from build123d import *

# Parameters (mm, degrees)
F1_DEPTH = 25


with BuildPart() as f1:
    # F0 (on Top) → F1 (new body)
    with BuildSketch(Plane.XY):
        with BuildLine():
            ThreePointArc((-37.094474, -66.332496), (-76, 0), (-37.094474, 66.332496))
            Line((-37.094474, 66.332496), (-37.094474, 82))
            ThreePointArc((-37.094474, 82), (-75.625732, 48.792916), (-90, 0))
            ThreePointArc((-90, 0), (-75.625732, -48.792916), (-37.094474, -82))
            Line((-37.094474, -82), (-37.094474, -66.332496))
        make_face()
        with BuildLine():
            ThreePointArc((-90, 0), (-75.625732, 48.792916), (-37.094474, 82))
            Line((-37.094474, 82), (-90, 82))
            Line((-90, 82), (-90, 0))
        make_face()
        with BuildLine():
            Line((-90, -82), (-37.094474, -82))
            ThreePointArc((-37.094474, -82), (-75.625732, -48.792916), (-90, 0))
            Line((-90, 0), (-90, -82))
        make_face()
    extrude(amount=F1_DEPTH)


solid = f1.part
Read the model definition and answer for the solid it produces. Units are mm, in the model's axes. Coordinates: 2 decimals unless noted, no trailing zeros. Order: outer loops, then holes, each group sorted by start corner. A loop starts at its lowest first (then second) coordinate and runs counter-clockwise, first axis right, second up. Notation, with made-up numbers: M 50.5,37 L 83.5,37 A23 ccw 83.5,73 Z; hole C 42,83.5 d7. An arc over 180 degrees is marked long. Put each result on its own line as item: value. Start each with the question number.
Item 1: Given pin 1 Ø5 at (y, z) = (43.5, 19) entering from +X; pin 2 Ø8 at (y, z) = (-57.5, 20) entering from +X, each flat-ended and moving along its own axis, determine where each tip first touches the part or whether it passes through.
Item 2: Section D-D, the plane y = -1 is taken. Determine the outline of the cut face in (x, z).
Item 3: Section B-B, the plane z = 16 is taken. Determine the outline of the cut face in (x, y), plus the area to 3 significant figures.
Item 4: Section C-C, the plane x = -42.5 is taken. Determine the outline of the cut face in (y, z).
Item 5: Section A-A, the plane x = -50 is taken. Determine the outline of the cut face in (y, z), plus the area to 3 significant figures.
Item 6: The mould has two halves that part along Y. Classify faces 1 (the face through (-37.094, -74, 12)), 2 (the face through (-75.99, -1.13, 12.32)), 3 (the face through (-63, 82, 12)), 4 (the face through (-64, -82, 12)): +Y half, -Y half, draft (parallel to the pull), parting line (faces both ways), or undercut.
Item 7: Consider probe 1 along Y at (x, z) = (-70, 13.25); probe 2 along Y at (x, z) = (-50.5, 11.75); probe 3 along X at (y, z) = (57.5, 24). Determine where each line is inside the solid, lowest interval first. Write a range as [from, to].
Computed:
1. pin 1: stops at x = -60.5
1. pin 2: stops at x = -44.65
2. outline: M -90,0 L -75.99,0 L -75.99,25 L -90,25 Z
3. outline: M -90,-82 L -37.09,-82 L -37.09,-66.33 A76 cw -37.09,66.33 L -37.09,82 L -90,82 Z
3. area: 5,010 mm2
4. outline: M -82,0 L -63.01,0 L -63.01,25 L -82,25 Z; M 63.01,0 L 82,0 L 82,25 L 63.01,25 Z
5. outline: M -82,0 L -57.24,0 L -57.24,25 L -82,25 Z; M 57.24,0 L 82,0 L 82,25 L 57.24,25 Z
5. area: 1,240 mm2
6. face 1: draft
6. face 2: undercut
6. face 3: +Y half
6. face 4: -Y half
7. probe 1: y = [-82, -29.6], [29.6, 82]
7. probe 2: y = [-82, -56.8], [56.8, 82]
7. probe 3: x = [-90, -49.7]
